from build123d import *

# Parameters (mm, degrees)
BOX_W        = 30
BOX_H        = 30
BOX_DEPTH    = 10
BOX001_W     = 26
BOX001_H     = 26
BOX001_DEPTH = 8


with BuildPart() as part:
    # Box → Box (join)
    with BuildSketch(Plane.XY):
        with Locations((15, 15)):
            Rectangle(BOX_W, BOX_H)
    extrude(amount=BOX_DEPTH)

    # Box001 → Box001 (cut)
    with BuildSketch(Plane(origin=(2, 2, 2), x_dir=(1, 0, 0), z_dir=(0, 0, 1))):
        with Locations((13, 13)):
            Rectangle(BOX001_W, BOX001_H)
    extrude(amount=BOX001_DEPTH, mode=Mode.SUBTRACT)


solid = part.part
Geometry: final body of the model. Coordinates: model frame, mm. A direction names the side the tool comes from. Give positions to 0.01 mm unless a question says otherwise; leave off trailing zeros. Write each loop counter-clockwise with the first axis right and the second up, starting at its lowest first coordinate (ties: lowest second). Pieces come first, ordered by that corner, then holes.
(1) Access query for faces 1 (the flat face through (0, 15, 5)), 2 (the flat face through (2, 15, 6)). Directions: +Z, -Z, +X, -X, +Y, -Y. A direction counts if a zero-diameter tool reaches every point of the face in a straight line with its end or side. Return the directions, or none.
(2) First-contact query: P1, Ø10, axis at x = 21, y = 8.5, coming from the +Z side. Flat tip, straight axial feed; report the tip coordinate or a pass-through.
(3) Cut plane B-B, the plane x = 9.75. Return loops of the section in (y, z).
(4) Mould query, pull axis X, two halves, no side actions, for faces 3 (the flat face through (15, 0, 5)), 4 (the flat face through (28, 15, 6)), 5 (the flat face through (30, 15, 5)). Classes: released by +X, released by -X, zero draft, split by the parting line, or undercut.
(5) Cut plane A-A, the plane z = 4.25. Return loops of the section in (x, y).
(6) Ray query, line 1 (X direction, y = 27.25, z = 2.75); line 2 (Z direction, x = 19.75, y = 7.5). Return the intervals inside material, ascending.
Values follow:
1. face 1: +Z, -Z, -X, +Y, -Y
1. face 2: +Z
2. P1: stops at z = 2
3. outline: (0, 0) - (30, 0) - (30, 10) - (28, 10) - (28, 2) - (2, 2) - (2, 10) - (0, 10) - close
4. face 3: zero draft
4. face 4: undercut
4. face 5: released by +X
5. outline: (0, 0) - (30, 0) - (30, 30) - (0, 30) - close; hole (2, 2) - (28, 2) - (28, 28) - (2, 28) - close
6. line 1: x = 0 to 2, 28 to 30
6. line 2: z = 0 to 2
